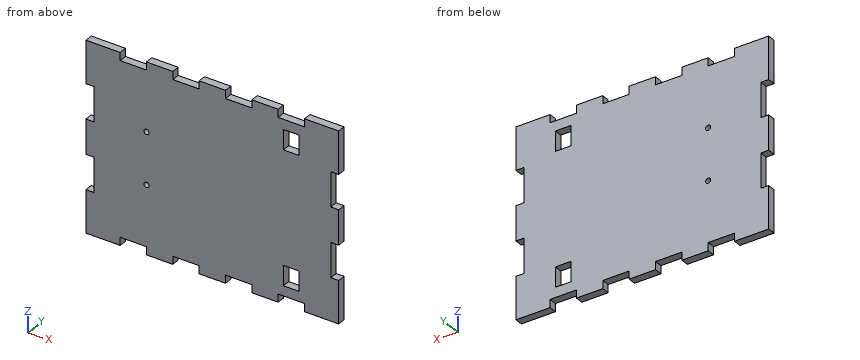
from build123d import *

# Parameters (mm, degrees)
SKETCH2_R           = 1.9
SKETCH2_R_2         = 1.95
SKETCH2_W           = 12
SKETCH2_H           = 15
BOSS_EXTRUDE2_DEPTH = 6


with BuildPart() as part:
    # Sketch2 → Boss-Extrude2 (new body)
    with BuildSketch(Plane(origin=(0, 0, 0), x_dir=(1, 0, 0), z_dir=(0, 1, 0))):
        Polygon((203.50455835, 73.988552732), (223.50455835, 73.988552732), (223.50455835, 67.988552732), (243.50455835, 67.988552732), (243.50455835, 73.988552732), (263.50455835, 73.988552732), (263.50455835, 67.988552732), (283.50455835, 67.988552732), (283.50455835, 73.988552732), (309.50455835, 73.988552732), (309.50455835, 41.988552732), (303.50455835, 41.988552732), (303.50455835, 15.988552732), (309.50455835, 15.988552732), (309.50455835, -10.011447268), (303.50455835, -10.011447268), (303.50455835, -36.011447268), (309.50455835, -36.011447268), (309.50455835, -68.011447268), (283.50455835, -68.011447268), (283.50455835, -62.011447268), (263.50455835, -62.011447268), (263.50455835, -68.011447268), (243.50455835, -68.011447268), (243.50455835, -62.011447268), (223.50455835, -62.011447268), (223.50455835, -68.011447268), (203.50455835, -68.011447268), (203.50455835, -62.011447268), (183.50455835, -62.011447268), (183.50455835, -68.011447268), (163.50455835, -68.011447268), (163.50455835, -62.011447268), (143.50455835, -62.011447268), (143.50455835, -68.011447268), (117.50455835, -68.011447268), (117.50455835, -36.011447268), (123.50455835, -36.011447268), (123.50455835, -10.011447268), (117.50455835, -10.011447268), (117.50455835, 15.988552732), (123.50455835, 15.988552732), (123.50455835, 41.988552732), (117.50455835, 41.988552732), (117.50455835, 73.988552732), (143.50455835, 73.988552732), (143.50455835, 67.988552732), (163.50455835, 67.988552732), (163.50455835, 73.988552732), (183.50455835, 73.988552732), (183.50455835, 67.988552732), (203.50455835, 67.988552732), align=None)
        with Locations(Location((163.50455835, 22.488552732, 0), (0, 0, 270))):
            Circle(SKETCH2_R, mode=Mode.SUBTRACT)
        with Locations(Location((163.50455835, -16.511447268, 0), (0, 0, 270))):
            Circle(SKETCH2_R_2, mode=Mode.SUBTRACT)
        with Locations((273.50455835, -47.011447268)):
            Rectangle(SKETCH2_W, SKETCH2_H, mode=Mode.SUBTRACT)
        with Locations((273.50455835, 52.988552732)):
            Rectangle(SKETCH2_W, SKETCH2_H, mode=Mode.SUBTRACT)
    extrude(amount=BOSS_EXTRUDE2_DEPTH)


solid = part.part
Build history of the part. All positions in model axes, mm. Round coordinates to 2 decimals unless told otherwise and drop trailing zeros. Write each loop counter-clockwise with the first axis right and the second up, starting at its lowest first coordinate (ties: lowest second). Pieces come first, ordered by that corner, then holes. Notation, with made-up numbers: (37.5, 3) -> (56.5, 3) arc R8 ccw to (56.5, 16) -> close; hole circle Ø10 at (-15.5, -39.5). An arc over 180 degrees is marked (long way). Write item = value, one per line.
(1) Band-saw the part on D-D (x = 153). Give the cut face in (y, z), then the cut area to 3 significant figures.
Answer:
outline = (0, -67.99) -> (6, -67.99) -> (6, 62.01) -> (0, 62.01) -> close
area = 780 mm2
(2) Band-saw the part on B-B (z = -50). Give the cut face in (x, y), then the cut area to 3 significant figures.
Answer:
outline = (117.5, 0) -> (267.5, 0) -> (267.5, 6) -> (117.5, 6) -> close; (279.5, 0) -> (309.5, 0) -> (309.5, 6) -> (279.5, 6) -> close
area = 1,080 mm2
(3) Band-saw the part on C-C (y = 1.4). State how many separate pieces and enclosed holes the cut face has, then the cut area to 3 significant figures.
Answer:
separate_pieces = 1
enclosed_holes = 4
area = 25,300 mm2
(4) Band-saw the part on A-A (x = 269.5). Give the cut face in (y, z), then the cut area to 3 significant figures.
Answer:
outline = (0, -67.99) -> (6, -67.99) -> (6, -60.49) -> (0, -60.49) -> close; (0, -45.49) -> (6, -45.49) -> (6, 39.51) -> (0, 39.51) -> close; (0, 54.51) -> (6, 54.51) -> (6, 62.01) -> (0, 62.01) -> close
area = 600 mm2
(5) Flat gauge pin, fed straight in: pin 1 (1 mm diameter, centred on x = 277.5, y = 3, fed in from -Z). Where does the tip first touch, or does it go through?
Answer:
pin_1 = -67.99
(6) Probe L1, parallel to Z at x = 268.5, y = 5.05; L2, parallel to X at y = 3.95, z = 32.5; L3, parallel to Z at x = 234, y = 1.5. List the from-to ranges inside material, lowest first.
Answer:
L1 = -67.99 to -60.49, -45.49 to 39.51, 54.51 to 62.01
L2 = 123.5 to 303.5
L3 = -67.99 to 62.01
